from build123d import *

# Parameters (mm, degrees)
SKETCH3_R                = 10
SKETCH3_R_2              = 6.5
BOSS_EXTRUDE1_DEPTH      = 1.1
BOSS_EXTRUDE1_DEPTH_BACK = 1.1
FILLET1_R                = 0.22
FILLET2_R                = 0.1


with BuildPart() as part:
    # Sketch3 → Boss-Extrude1 (new body, two sides)
    with BuildSketch(Plane.XY) as boss_extrude1_sk:
        Circle(SKETCH3_R)
        Circle(SKETCH3_R_2, mode=Mode.SUBTRACT)
    extrude(amount=BOSS_EXTRUDE1_DEPTH)
    extrude(boss_extrude1_sk.sketch, amount=-BOSS_EXTRUDE1_DEPTH_BACK)

    # Fillet1
    fillet1_edges = [part.edges().sort_by_distance(p)[0] for p in [
        (-10, 0, 1.1),
        (-6.5, 0, 1.1),
    ]]
    fillet(fillet1_edges, radius=FILLET1_R)

    # Fillet2
    fillet2_edges = [part.edges().sort_by_distance(p)[0] for p in [
        (-10, 0, -1.1),
        (-6.5, 0, -1.1),
    ]]
    fillet(fillet2_edges, radius=FILLET2_R)


solid = part.part
Source: CAD feature listing. Evaluate the final solid. Frame: model axes, mm. Round coordinates to 2 decimals unless told otherwise and drop trailing zeros. Loops run counter-clockwise (first coordinate to the right, second up) from the corner with the lowest first, then second, coordinate; pieces in that order, holes last. Notation, with made-up numbers: (37, 88.5) -> (78, 88.5) arc R15 ccw to (78, 108.5) -> close; hole circle Ø9 at (68.5, 36). An arc over 180 degrees is marked (long way). Answer as a JSON object with one key per item and string values. Group by question number.
Q1. Section query A-A (y = 0). Output: boundary loops of the cut face in (x, z), plus the area to 3 significant figures.
Q2. Ray query, line 1 (Y direction, x = 0, z = 0.4); line 2 (X direction, y = 3.25, z = 0.75); line 3 (Y direction, x = -4.5, z = 0.6). Return the intervals inside material, ascending. Write a range as from..to.
Q3. Section query C-C (z = 0.55). Output: boundary loops of the cut face in (x, y), plus the area to 3 significant figures.
Q4. Contact query for flat-ended pins moving along their axis: P1, Ø1, axis at y = -3.5, z = -0.5, coming from the -X side; P2, Ø5, axis at x = -4.5, y = 4.5, coming from the +Z side; P3, Ø11.5, axis at x = 0, y = 0, coming from the +Z side. Output: stop coordinate, or through.
Completed:
{
 "1": {"outline": "(-10, -1) arc R0.1 ccw to (-9.9, -1.1) -> (-6.6, -1.1) arc R0.1 ccw to (-6.5, -1) -> (-6.5, 0.88) arc R0.22 ccw to (-6.72, 1.1) -> (-9.78, 1.1) arc R0.22 ccw to (-10, 0.88) -> close; (6.5, -1) arc R0.1 ccw to (6.6, -1.1) -> (9.9, -1.1) arc R0.1 ccw to (10, -1) -> (10, 0.88) arc R0.22 ccw to (9.78, 1.1) -> (6.72, 1.1) arc R0.22 ccw to (6.5, 0.88) -> close", "area": "15.3 mm²"},
 "2": {"line 1": "-10..-6.5, 6.5..10", "line 2": "-9.46..-5.63, 5.63..9.46", "line 3": "-8.93..-4.69, 4.69..8.93"},
 "3": {"outline": "circle Ø20 at (0, 0); hole circle Ø13 at (0, 0)", "area": "181 mm²"},
 "4": {"P1": "x = -9.54", "P2": "z = 1.1", "P3": "through"}
}
